from build123d import *

# Parameters (mm, degrees)
SKETCH1_W           = 15
SKETCH1_H           = 15
SKETCH1_W_2         = 12
SKETCH1_H_2         = 12
BOSS_EXTRUDE1_DEPTH = 110


with BuildPart() as part:
    # Sketch1 → Boss-Extrude1 (new body, symmetric)
    with BuildSketch(Plane(origin=(0, 0, 0), x_dir=(0, 0, -1), z_dir=(1, 0, 0))):
        Rectangle(SKETCH1_W, SKETCH1_H)
        Rectangle(SKETCH1_W_2, SKETCH1_H_2, mode=Mode.SUBTRACT)
    extrude(amount=BOSS_EXTRUDE1_DEPTH, both=True)


solid = part.part
For this review, take the finished solid that the model builds, in its own axes (mm). A direction names the side the tool comes from. Give positions to 0.01 mm unless a question says otherwise; leave off trailing zeros. Loops run counter-clockwise (first coordinate to the right, second up) from the corner with the lowest first, then second, coordinate; pieces in that order, holes last.
Item 1: Take a section at A-A, the plane y = 1.5. State the section outline as (x, z) points, and give its area (3 significant figures).
Item 2: Draft analysis for pull direction Z (two halves, no side actions). For faces 1 (the flat face through (2, -6, 0)), 2 (the flat face through (2, 0, 7.5)), 3 (the flat face through (2, -7.5, 0)), state which applies: +Z half, -Z half, draft (parallel to the pull), parting line (faces both ways), or undercut.
Item 3: For line 1 along Y through (x, z) = (31, -2.75), list the stretches that pass through material, from the lowest coordinate up.
Item 4: Take a section at B-B, the plane x = -55. State the section outline as (y, z) points.
Item 5: Insertion check: pin 1 (4 mm diameter, centred on y = -2.5, z = -1.5, fed in from -X). The pin has a flat end and moves straight along its axis. Give the tip position at first contact, or say it passes through.
Item 6: Tool access review of faces 4 (the flat face through (2, 0, -7.5)), 5 (the flat face through (2, 0, -6)): name each direction out of +Z, -Z, +X, -X, +Y, -Y from which nothing blocks a thin tool from reaching the whole face with its end or side.
Calculated:
1. outline: (-110, -7.5) - (110, -7.5) - (110, -6) - (-110, -6) - close; (-110, 6) - (110, 6) - (110, 7.5) - (-110, 7.5) - close
1. area: 660 mm2
2. face 1: undercut
2. face 2: +Z half
2. face 3: draft
3. line 1: y = -7.5 to -6, 6 to 7.5
4. outline: (-7.5, -7.5) - (7.5, -7.5) - (7.5, 7.5) - (-7.5, 7.5) - close; hole (-6, -6) - (6, -6) - (6, 6) - (-6, 6) - close
5. pin 1: passes through
6. face 4: -Z, +X, -X, +Y, -Y
6. face 5: +X, -X
